Geometry: final body of the model. Coordinates: model frame, mm. Face numbers are marked on the shaded views. A direction names the side the tool comes from. Round coordinates to 2 decimals unless told otherwise and drop trailing zeros. Loops run counter-clockwise (first coordinate to the right, second up) from the corner with the lowest first, then second, coordinate; pieces in that order, holes last. Notation, with made-up numbers: M -39.75,-35.75 L 14.25,-35.75 A20 cw 14.25,0.25 Z; hole C -10,25 d11. An arc over 180 degrees is marked long. Answer as a JSON object with one key per item and string values.
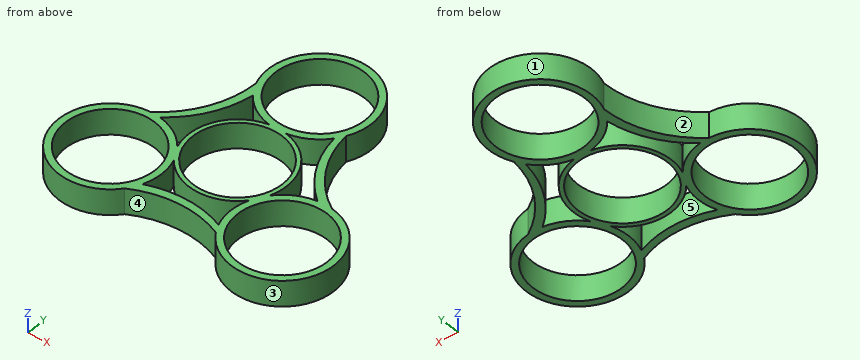
```python
from build123d import *

# Parameters (mm, degrees)
F0_R     = 11.049
F1_DEPTH = 6.35


with BuildPart() as f1:
    # F0 (on Top) → F1 (new body)
    with BuildSketch(Plane.XY):
        with BuildLine():
            ThreePointArc((-11.771514, 19.656815), (-14.475948, 8.897779), (-21.697628, 0.476489))
            ThreePointArc((-21.697628, 0.476489), (-32.441402, -18.027731), (-11.137544, -20.022838))
            ThreePointArc((-11.137544, -20.022838), (-0.467729, -16.985428), (10.436163, -19.028942))
            ThreePointArc((10.436163, -19.028942), (31.833175, -19.081213), (22.909058, 0.366023))
            ThreePointArc((22.909058, 0.366023), (14.943677, 8.087649), (11.261466, 18.552453))
            ThreePointArc((11.261466, 18.552453), (0.608228, 37.108944), (-11.771514, 19.656815))
        make_face()
        with Locations((-21.151386, -12.211759)):
            Circle(F0_R, mode=Mode.SUBTRACT)
        with BuildLine():
            ThreePointArc((-9.272628, -7.718977), (0, -12.065), (9.272628, -7.718977))
            ThreePointArc((9.272628, -7.718977), (8.452064, -12.342974), (9.367997, -16.949029))
            ThreePointArc((9.367997, -16.949029), (0.017693, -15.074095), (-9.344314, -16.889691))
            ThreePointArc((-9.344314, -16.889691), (-8.451774, -12.31103), (-9.272628, -7.718977))
        make_face(mode=Mode.SUBTRACT)
        with Locations((21.151386, -12.211759)):
            Circle(F0_R, mode=Mode.SUBTRACT)
        Circle(F0_R, mode=Mode.SUBTRACT)
        with BuildLine():
            ThreePointArc((-9.954744, 16.537259), (-6.435778, 13.474967), (-2.048516, 11.889819))
            ThreePointArc((-2.048516, 11.889819), (-10.448596, 6.0325), (-11.321144, -4.170843))
            ThreePointArc((-11.321144, -4.170843), (-14.915361, -1.148215), (-19.362288, 0.361591))
            ThreePointArc((-19.362288, 0.361591), (-13.063396, 7.521725), (-9.954744, 16.537259))
        make_face(mode=Mode.SUBTRACT)
        with BuildLine():
            ThreePointArc((11.321144, -4.170843), (10.448596, 6.0325), (2.048516, 11.889819))
            ThreePointArc((2.048516, 11.889819), (6.463297, 13.491189), (9.994291, 16.587438))
            ThreePointArc((9.994291, 16.587438), (13.045703, 7.55237), (19.299058, 0.352432))
            ThreePointArc((19.299058, 0.352432), (14.887552, -1.163936), (11.321144, -4.170843))
        make_face(mode=Mode.SUBTRACT)
        with Locations((0, 24.423517)):
            Circle(F0_R, mode=Mode.SUBTRACT)
    extrude(amount=F1_DEPTH)


solid = f1.part
```
1) Set-up query: the marked faces 1 and 2. Return all of +Z, -Z, +X, -X, +Y, -Y with unobstructed straight access to the full face (end or side cutting, diameter ignored); none if empty.
Geometry results:
{"face 1": "+Z, -Z", "face 2": "+Z, -Z, -X"}
2) Cut plane D-D on z = 1. Return the cut outline in (x, y) (3 decimals).
Geometry results:
{"outline": "M -21.698,0.476 A12.7 ccw long -11.138,-20.023 A24.196 cw 10.436,-19.029 A12.7 ccw long 22.909,0.366 A24.196 cw 11.261,18.552 A12.7 ccw long -11.772,19.657 A24.196 cw Z; hole C -21.151,-12.212 d22.098; hole M -19.362,0.362 A12.7 cw -11.321,-4.171 A12.065 cw -2.049,11.89 A12.7 cw -9.955,16.537 A24.642 cw Z; hole C 0,0 d22.098; hole C 0,24.424 d22.098; hole M -9.344,-16.89 A24.642 cw 9.368,-16.949 A12.7 cw 9.273,-7.719 A12.065 cw -9.273,-7.719 A12.7 cw Z; hole M 2.049,11.89 A12.065 cw 11.321,-4.171 A12.7 cw 19.299,0.352 A24.642 cw 9.994,16.587 A12.7 cw Z; hole C 21.151,-12.212 d22.098"}
3) Cut plane C-C on x = 0. Return the cut outline in (y, z) (3 decimals), and give its area (3 significant figures).
Geometry results:
{"outline": "M -16.968,0 L -15.074,0 L -15.074,6.35 L -16.968,6.35 Z; M -12.065,0 L -11.049,0 L -11.049,6.35 L -12.065,6.35 Z; M 11.049,0 L 13.375,0 L 13.375,6.35 L 11.049,6.35 Z; M 35.473,0 L 37.124,0 L 37.124,6.35 L 35.473,6.35 Z", "area": "43.7 mm2"}
4) Cut plane A-A on x = 20.5. Return the cut outline in (y, z), and give its area (3 significant figures).
Geometry results:
{"outline": "M -24.9,0 L -23.24,0 L -23.24,6.35 L -24.9,6.35 Z; M -1.18,0 L 2.01,0 L 2.01,6.35 L -1.18,6.35 Z", "area": "30.8 mm2"}
5) Line query: probe 1 along Y at (x, z) = (0, 2) (3 decimals); probe 2 along Y at (x, z) = (13, 6); probe 3 along Y at (x, z) = (16, 1). Output: solid intervals per line, ascending.
Geometry results:
{"probe 1": "-16.968 to -15.074, -12.065 to -11.049, 11.049 to 13.375, 35.473 to 37.124", "probe 2": "-21.95 to -19.67, -4.75 to -2.47, 7.63 to 11.79", "probe 3": "-23.82 to -21.99, -2.44 to -0.6, 3.44 to 6.57"}
6) Pull-direction query (Y, two-part tool) for the marked faces 3, 4 and 5; classes: +Y half, -Y half, draft (parallel to the pull), parting line (faces both ways), or undercut.
Geometry results:
{"face 3": "parting line", "face 4": "-Y half", "face 5": "undercut"}
7) Cut plane B-B on y = 6. Return the cut outline in (x, z), and give its area (3 significant figures).
Geometry results:
{"outline": "M -16.24,0 L -14.02,0 L -14.02,6.35 L -16.24,6.35 Z; M -10.47,0 L -9.28,0 L -9.28,6.35 L -10.47,6.35 Z; M 9.28,0 L 10.47,0 L 10.47,6.35 L 9.28,6.35 Z; M 14.01,0 L 16.44,0 L 16.44,6.35 L 14.01,6.35 Z", "area": "44.6 mm2"}
8) First-contact query: pin 1 (2 mm diameter, centred on x = 20.5, z = 4, fed in from -Y); pin 2 (3 mm diameter, centred on y = 7.5, z = 1.5, fed in from +X); pin 3 (1 mm diameter, centred on x = -9.5, z = 5, fed in from -Y); pin 4 (1.5 mm diameter, centred on y = -7.5, z = 5, fed in from -X). Flat tips, straight axial feed; report the tip coordinate or a pass-through.
Geometry results:
{"pin 1": "y = -24.91", "pin 2": "x = 16.44", "pin 3": "y = -19.43", "pin 4": "x = -33.22"}
